Geometry: final body of the model. Coordinates: model frame, mm. A direction names the side the tool comes from. Coordinates: 2 decimals unless noted, no trailing zeros. Order: outer loops, then holes, each group sorted by start corner. A loop starts at its lowest first (then second) coordinate and runs counter-clockwise, first axis right, second up. Notation, with made-up numbers: (23.25, 48) - (53.25, 48) arc R17 cw to (53.25, 72) - close; hole circle Ø11 at (68.25, -19). An arc over 180 degrees is marked (long way). Use one line per item in the form item = value. Start each with the question number.
```python
from build123d import *

# Parameters (mm, degrees)
BOSS_EXTRUDE1_DEPTH                        = 10
BOSS_EXTRUDE2_START                        = 10
SKETCH4_R                                  = 4
BOSS_EXTRUDE2_DEPTH                        = 1
BOSS_EXTRUDE4_START                        = 11.5
BOSS_EXTRUDE4_DEPTH                        = 7
CUT_EXTRUDE2_START                         = 11.5
CUT_EXTRUDE2_DEPTH                         = 7
BOSS_EXTRUDE3_START                        = 10
BOSS_EXTRUDE3_DEPTH                        = 1.5
MIRROR4_DEPTH                              = 8
MIRROR4_START                              = 8
MIRROR4_2_DEPTH                            = 2
MIRROR4_START_2                            = 10
MIRROR4_3_DEPTH                            = 1.5
MIRROR4_4_DEPTH                            = 3
MIRROR4_START_3                            = -11.5
MIRROR4_5_DEPTH                            = 7
MIRROR4_START_4                            = 4.5
MIRROR4_6_DEPTH                            = 7
SKETCH2_R                                  = 4.5
SKETCH2_W                                  = 40
SKETCH2_H                                  = 10
CUT_EXTRUDE1_DEPTH                         = 5
BOSS_EXTRUDE5_START                        = 10
BOSS_EXTRUDE5_DEPTH                        = 50
SKETCH8_R                                  = 1.35
CUT_EXTRUDE3_DEPTH                         = 4
SKETCH9_R                                  = 1.35
CUT_EXTRUDE4_DEPTH                         = 4
MIRROR5_AT_THE_SECOND_PLANE_COPY_1_SKETC_R = 1.35
MIRROR5_AT_THE_SECOND_PLANE_COPY_1_DEPTH   = 4


with BuildPart() as part:
    # Sketch3 → Boss-Extrude1 (new body)
    with BuildSketch(Plane(origin=(0, 0, 0), x_dir=(1, 0, 0), z_dir=(0, 1, 0))):
        with BuildLine():
            Line((-41, 0), (-41, -12.5))
            ThreePointArc((-41, -12.5), (-39.242640687, -16.742640687), (-35, -18.5))
            Line((-35, -18.5), (0, -18.5))
            Line((0, -18.5), (0, 0))
            Line((0, 0), (-41, 0))
        make_face()
    extrude(amount=BOSS_EXTRUDE1_DEPTH)

    # Sketch4 → Boss-Extrude2 (add)
    with BuildSketch(Plane(origin=(0, 0, 0), x_dir=(1, 0, 0), z_dir=(0, 1, 0)).offset(BOSS_EXTRUDE2_START)):
        with Locations((-30, -8)):
            Circle(SKETCH4_R)
        with BuildLine():
            Line((-26, -4.5), (-28.063508327, -4.5))
            ThreePointArc((-28.063508327, -4.5), (-26.554280431, -5.968493994), (-26, -8))
            Line((-26, -8), (-26, -4.5))
        make_face()
        with BuildLine():
            Line((-26, -11.5), (-26, -8))
            ThreePointArc((-26, -8), (-26.554280431, -10.031506006), (-28.063508327, -11.5))
            Line((-28.063508327, -11.5), (-26, -11.5))
        make_face()
    extrude(amount=BOSS_EXTRUDE2_DEPTH)

    # Sketch6 → Boss-Extrude4 (add)
    with BuildSketch(Plane.XY.offset(BOSS_EXTRUDE4_START)):
        Polygon((-23.252522581, 10), (-26, 11), (-26, 10), align=None)
    extrude(amount=-BOSS_EXTRUDE4_DEPTH)

    # Sketch6<3> → Cut-Extrude2 (cut)
    with BuildSketch(Plane.XY.offset(CUT_EXTRUDE2_START)):
        with BuildLine():
            Line((-20.32871818, 10), (-23.252522581, 10))
            Line((-23.252522581, 10), (-19.414499368, 8.603073792))
            ThreePointArc((-19.414499368, 8.603073792), (-17.730779711, 8.15192247), (-15.994297935, 8))
            Line((-15.994297935, 8), (0, 8))
            Line((0, 8), (0, 9))
            Line((0, 9), (-15.994297935, 9))
            ThreePointArc((-15.994297935, 9), (-17.557131534, 9.136730223), (-19.072479224, 9.542766413))
            Line((-19.072479224, 9.542766413), (-20.32871818, 10))
        make_face()
    extrude(amount=-CUT_EXTRUDE2_DEPTH, mode=Mode.SUBTRACT)

    # Sketch4<3> → Boss-Extrude3 (add)
    with BuildSketch(Plane(origin=(0, 0, 0), x_dir=(1, 0, 0), z_dir=(0, 1, 0)).offset(BOSS_EXTRUDE3_START)):
        with BuildLine():
            ThreePointArc((-28.063508327, -11.5), (-34, -8), (-28.063508327, -4.5))
            Line((-28.063508327, -4.5), (-26, -4.5))
            Line((-26, -4.5), (-25.126602828, -4.5))
            ThreePointArc((-25.126602828, -4.5), (-36, -8), (-25.126602828, -11.5))
            Line((-25.126602828, -11.5), (-26, -11.5))
            Line((-26, -11.5), (-28.063508327, -11.5))
        make_face()
    extrude(amount=BOSS_EXTRUDE3_DEPTH)

    # Mirror4: read off the stored shape, not the designer's step
    # Mirror4 outline → Mirror4 (add)
    with BuildSketch(Plane(origin=(0, 0, 0), x_dir=(1, 0, 0), z_dir=(0, 1, 0))):
        with BuildLine():
            Line((0, -18.5), (35, -18.5))
            ThreePointArc((35, -18.5), (39.242640687, -16.742640687), (41, -12.5))
            Line((41, -12.5), (41, 12.5))
            ThreePointArc((41, 12.5), (39.242640687, 16.742640687), (35, 18.5))
            Line((35, 18.5), (-35, 18.5))
            ThreePointArc((-35, 18.5), (-39.242640687, 16.742640687), (-41, 12.5))
            Line((-41, 12.5), (-41, 0))
            Line((-41, 0), (0, 0))
            Line((0, 0), (0, -18.5))
        make_face()
    extrude(amount=MIRROR4_DEPTH)

    # Mirror4 2 outline → Mirror4 2 (add)
    with BuildSketch(Plane(origin=(0, 0, 0), x_dir=(1, 0, 0), z_dir=(0, 1, 0)).offset(MIRROR4_START)):
        with BuildLine():
            Line((0, -11.5), (0, -18.5))
            Line((0, -18.5), (35, -18.5))
            ThreePointArc((35, -18.5), (39.242640687, -16.742640687), (41, -12.5))
            Line((41, -12.5), (41, 12.5))
            ThreePointArc((41, 12.5), (39.242640687, 16.742640687), (35, 18.5))
            Line((35, 18.5), (-35, 18.5))
            ThreePointArc((-35, 18.5), (-39.242640687, 16.742640687), (-41, 12.5))
            Line((-41, 12.5), (-41, 0))
            Line((-41, 0), (0, 0))
            Line((0, 0), (0, -4.5))
            Line((0, -4.5), (28.063508327, -4.5))
            ThreePointArc((28.063508327, -4.5), (34, -8), (28.063508327, -11.5))
            Line((28.063508327, -11.5), (0, -11.5))
        make_face()
        with BuildLine():
            ThreePointArc((28.063508327, 11.5), (34, 8), (28.063508327, 4.5))
            Line((28.063508327, 4.5), (-28.063508327, 4.5))
            ThreePointArc((-28.063508327, 4.5), (-34, 8), (-28.063508327, 11.5))
            Line((-28.063508327, 11.5), (28.063508327, 11.5))
        make_face(mode=Mode.SUBTRACT)
    extrude(amount=MIRROR4_2_DEPTH)

    # Mirror4 3 outline → Mirror4 3 (add)
    with BuildSketch(Plane(origin=(0, 0, 0), x_dir=(1, 0, 0), z_dir=(0, 1, 0)).offset(MIRROR4_START_2)):
        with BuildLine():
            Line((28.063508327, -11.5), (25.126602828, -11.5))
            ThreePointArc((25.126602828, -11.5), (36, -8), (25.126602828, -4.5))
            Line((25.126602828, -4.5), (28.063508327, -4.5))
            ThreePointArc((28.063508327, -4.5), (34, -8), (28.063508327, -11.5))
        make_face()
        with BuildLine():
            Line((-28.063508327, 11.5), (-25.126602828, 11.5))
            ThreePointArc((-25.126602828, 11.5), (-36, 8), (-25.126602828, 4.5))
            Line((-25.126602828, 4.5), (-28.063508327, 4.5))
            ThreePointArc((-28.063508327, 4.5), (-34, 8), (-28.063508327, 11.5))
        make_face()
        with BuildLine():
            ThreePointArc((25.126602828, 4.5), (36, 8), (25.126602828, 11.5))
            Line((25.126602828, 11.5), (28.063508327, 11.5))
            ThreePointArc((28.063508327, 11.5), (34, 8), (28.063508327, 4.5))
            Line((28.063508327, 4.5), (25.126602828, 4.5))
        make_face()
    extrude(amount=MIRROR4_3_DEPTH)

    # Mirror4 4 outline → Mirror4 4 (add)
    with BuildSketch(Plane(origin=(0, 0, 0), x_dir=(1, 0, 0), z_dir=(0, 1, 0)).offset(MIRROR4_START)):
        with BuildLine():
            Line((0, -11.5), (28.063508327, -11.5))
            ThreePointArc((28.063508327, -11.5), (34, -8), (28.063508327, -4.5))
            Line((28.063508327, -4.5), (0, -4.5))
            Line((0, -4.5), (0, -11.5))
        make_face()
        with BuildLine():
            Line((28.063508327, 11.5), (-28.063508327, 11.5))
            ThreePointArc((-28.063508327, 11.5), (-34, 8), (-28.063508327, 4.5))
            Line((-28.063508327, 4.5), (28.063508327, 4.5))
            ThreePointArc((28.063508327, 4.5), (34, 8), (28.063508327, 11.5))
        make_face()
    extrude(amount=MIRROR4_4_DEPTH)

    # Mirror4 5 outline → Mirror4 5 (cut)
    with BuildSketch(Plane.XY.offset(MIRROR4_START_3)):
        with BuildLine():
            Line((26, 11), (-26, 11))
            Line((-26, 11), (-19.414499368, 8.603073792))
            ThreePointArc((-19.414499368, 8.603073792), (-17.730779711, 8.15192247), (-15.994297935, 8))
            Line((-15.994297935, 8), (15.994297935, 8))
            ThreePointArc((15.994297935, 8), (17.730779711, 8.15192247), (19.414499368, 8.603073792))
            Line((19.414499368, 8.603073792), (26, 11))
        make_face()
        with BuildLine():
            Line((20.32871818, 10), (19.072479224, 9.542766413))
            ThreePointArc((19.072479224, 9.542766413), (17.557131534, 9.136730223), (15.994297935, 9))
            Line((15.994297935, 9), (-15.994297935, 9))
            ThreePointArc((-15.994297935, 9), (-17.557131534, 9.136730223), (-19.072479224, 9.542766413))
            Line((-19.072479224, 9.542766413), (-20.32871818, 10))
            Line((-20.32871818, 10), (20.32871818, 10))
        make_face(mode=Mode.SUBTRACT)
    extrude(amount=MIRROR4_5_DEPTH, mode=Mode.SUBTRACT)

    # Mirror4 6 outline → Mirror4 6 (cut)
    with BuildSketch(Plane.XY.offset(MIRROR4_START_4)):
        with BuildLine():
            Line((0, 10), (20.32871818, 10))
            Line((20.32871818, 10), (19.072479224, 9.542766413))
            ThreePointArc((19.072479224, 9.542766413), (17.557131534, 9.136730223), (15.994297935, 9))
            Line((15.994297935, 9), (0, 9))
            Line((0, 9), (0, 8))
            Line((0, 8), (15.994297935, 8))
            ThreePointArc((15.994297935, 8), (17.730779711, 8.15192247), (19.414499368, 8.603073792))
            Line((19.414499368, 8.603073792), (26, 11))
            Line((26, 11), (0, 11))
            Line((0, 11), (0, 10))
        make_face()
    extrude(amount=MIRROR4_6_DEPTH, mode=Mode.SUBTRACT)

    # Sketch2 → Cut-Extrude1 (cut)
    with BuildSketch(Plane(origin=(0, 0, 0), x_dir=(1, 0, 0), z_dir=(0, 1, 0))):
        with Locations(Location((-30, 0, 0), (0, 0, 270))):
            Circle(SKETCH2_R)
        with Locations(Location((30, 0, 0), (0, 0, 270))):
            Circle(SKETCH2_R)
        Rectangle(SKETCH2_W, SKETCH2_H)
    extrude(amount=CUT_EXTRUDE1_DEPTH, mode=Mode.SUBTRACT)

    # Sketch7 → Boss-Extrude5 (add)
    with BuildSketch(Plane(origin=(0, 0, 0), x_dir=(1, 0, 0), z_dir=(0, 1, 0)).offset(BOSS_EXTRUDE5_START)):
        with BuildLine():
            Line((-8, -12), (8, -12))
            ThreePointArc((8, -12), (10.828427125, -10.828427125), (12, -8))
            Line((12, -8), (12, 8))
            ThreePointArc((12, 8), (10.828427125, 10.828427125), (8, 12))
            Line((8, 12), (-8, 12))
            ThreePointArc((-8, 12), (-10.828427125, 10.828427125), (-12, 8))
            Line((-12, 8), (-12, -8))
            ThreePointArc((-12, -8), (-10.828427125, -10.828427125), (-8, -12))
        make_face()
    extrude(amount=BOSS_EXTRUDE5_DEPTH)

    # Sketch8 → Cut-Extrude3 (cut)
    with BuildSketch(Plane(origin=(0, 60, 0), x_dir=(1, 0, 0), z_dir=(0, 1, 0))):
        with Locations(Location((-8.5, 8.5, 0), (0, 0, 270))):
            Circle(SKETCH8_R)
        with Locations(Location((-8.5, -8.5, 0), (0, 0, 270))):
            Circle(SKETCH8_R)
        with Locations(Location((8.5, 8.5, 0), (0, 0, 270))):
            Circle(SKETCH8_R)
        with Locations(Location((8.5, -8.5, 0), (0, 0, 270))):
            Circle(SKETCH8_R)
    extrude(amount=-CUT_EXTRUDE3_DEPTH, mode=Mode.SUBTRACT)

    # Sketch9 → Cut-Extrude4 (cut)
    with BuildSketch(Plane(origin=(0, 10, 0), x_dir=(1, 0, 0), z_dir=(0, 1, 0))):
        with Locations(Location((-36.36, 13.86, 0), (0, 0, 270))):
            Circle(SKETCH9_R)
    cut_extrude4 = extrude(amount=-CUT_EXTRUDE4_DEPTH, mode=Mode.SUBTRACT)

    # Mirror5: Cut-Extrude4 across plane
    add(cut_extrude4.mirror(Plane.XY), mode=Mode.SUBTRACT)

    # Mirror5 at the second plane: Cut-Extrude4 across plane
    add(cut_extrude4.mirror(Plane(origin=(0, 0, 0), x_dir=(0, 0, 1), z_dir=(1, 0, 0))), mode=Mode.SUBTRACT)

    # Mirror5 at the second plane copy 1 sketc → Mirror5 at the second plane copy 1 (cut)
    with BuildSketch(Plane(origin=(0, 10, 0), x_dir=(-1, 0, 0), z_dir=(0, 1, 0))):
        with Locations(Location((-36.36, 13.86, 0), (0, 0, 270))):
            Circle(MIRROR5_AT_THE_SECOND_PLANE_COPY_1_SKETC_R)
    extrude(amount=-MIRROR5_AT_THE_SECOND_PLANE_COPY_1_DEPTH, mode=Mode.SUBTRACT)


solid = part.part
```
(1) Cut plane C-C on z = 0. Return the cut outline in (x, y).
(2) Cut plane A-A on y = 4. Return the cut outline in (x, z), plus the area to 3 significant figures.
(3) Draft query along X for faces 3 (the flat face through (0, 8, -8)), 4 (the flat face through (0, 5, 18.5)), 5 (the flat face through (-1, 10, -13)). Return one class per face: released by +X, released by -X, zero draft, split by the parting line, or undercut.
(4) Material intervals for L1, parallel to Z at x = 30, y = 11.15; L2, parallel to X at y = 1.25, z = 0; L3, parallel to Y at x = -15, z = 9.5, sorted ascending. Write a range as from..to.
(5) Cut plane D-D on y = 29.5. Return the cut outline in (x, z), plus the area to 3 significant figures.
(6) Contact query for flat-ended pins moving along their axis: pin 1 Ø9 at (x, z) = (-31, -7) entering from +Y; pin 2 Ø1 at (x, z) = (31, -14.5) entering from +Y; pin 3 Ø8 at (x, y) = (-12, 53) entering from -Z. Output: stop coordinate, or through.
(7) Cut plane B-B on x = 13.5. Return the cut outline in (y, z), plus the area to 3 significant figures.
(8) Set-up query: faces 1 (the cylindrical face through (36, 11, -8)), 2 (the cylindrical face through (17.58, 9.14, 7.95)). Return all of +Z, -Z, +X, -X, +Y, -Y with unobstructed straight access to the full face (end or side cutting, diameter ignored); none if empty.
Check sheet entries:
q1.outline = (-41, 0) - (-34.5, 0) - (-34.5, 5) - (-25.5, 5) - (-25.5, 0) - (-20, 0) - (-20, 5) - (20, 5) - (20, 0) - (25.5, 0) - (25.5, 5) - (34.5, 5) - (34.5, 0) - (41, 0) - (41, 10) - (12, 10) - (12, 60) - (-12, 60) - (-12, 10) - (-41, 10) - close
q2.outline = (-41, -12.5) arc R6 ccw to (-35, -18.5) - (35, -18.5) arc R6 ccw to (41, -12.5) - (41, 12.5) arc R6 ccw to (35, 18.5) - (-35, 18.5) arc R6 ccw to (-41, 12.5) - close; hole circle Ø9 at (-30, 0); hole (-20, -5) - (20, -5) - (20, 5) - (-20, 5) - close; hole circle Ø9 at (30, 0)
q2.area = 2,480 mm^2
q3.face_3 = undercut
q3.face_4 = zero draft
q3.face_5 = undercut
q4.L1 = -14..-12, -4..-2, 2..4, 12..14
q4.L2 = -41..-34.5, -25.5..-20, 20..25.5, 34.5..41
q4.L3 = 0..8, 9..10
q5.outline = (-12, -8) arc R4 ccw to (-8, -12) - (8, -12) arc R4 ccw to (12, -8) - (12, 8) arc R4 ccw to (8, 12) - (-8, 12) arc R4 ccw to (-12, 8) - close
q5.area = 562 mm^2
q6.pin_1 = 11.5
q6.pin_2 = 10
q6.pin_3 = -12
q7.outline = (0, -18.5) - (10, -18.5) - (10, 18.5) - (0, 18.5) - (0, 5) - (5, 5) - (5, -5) - (0, -5) - close; hole (8, -11.5) - (9, -11.5) - (9, -4.5) - (8, -4.5) - close; hole (8, 4.5) - (9, 4.5) - (9, 11.5) - (8, 11.5) - close
q7.area = 306 mm^2
q8.face_1 = +Y
q8.face_2 = none
